Design review of the part shown in the three views and the two pictorial views. Dimensions are in mm from the part's minimum x, y and z. A direction names the side the tool comes from. Give positions to 0.01 mm unless a question says otherwise; leave off trailing zeros. Order: outer loops, then holes, each group sorted by start corner. A loop starts at its lowest first (then second) coordinate and runs counter-clockwise, first axis right, second up.
Item 1: Consider section D-D (z = 32.5). Give the boundary of the cut face in (x, y), plus the area to 3 significant figures.
Item 2: For probe 1 along X at (y, z) = (17, 41); probe 2 along Z at (x, y) = (9, 12.5); probe 3 along X at (y, z) = (16.25, 16), list the stretches that pass through material, from the lowest coordinate up.
Item 3: The part is to be moulded in two halves that separate along Z. For the marked faces 1, 2, 3 and 4, say which applies: released by +Z, released by -Z, zero draft, split by the parting line, or undercut.
Item 4: Machinability: for the marked faces 5, 6, 7 and 8, which of the approach directions +Z, -Z, +X, -X, +Y, -Y give a long, thin tool a straight path to every point of the face, cutting with its end or side? Answer none if there is none.
Item 5: For P1, Ø5, axis at x = 43, y = 2, coming from the -Z side; P2, Ø6, axis at y = 8.5, z = 53.5, coming from the +X side; P3, Ø3, axis at x = 6.5, z = 18, coming from the -Y side; P4, Ø6, axis at y = 9, z = 29.5, coming from the -X side, all flat-tipped, find the tip position at first contact; note any pin that passes through.
Item 6: Consider section C-C (x = 7.5). Give the boundary of the cut face in (y, z), plus the area to 3 significant figures.
Item 7: Consider section A-A (y = 7.5). Give the number of separate pieces and of enclosed holes in the cut face, plus the area to 4 significant figures.
Item 8: Consider section B-B (z = 44). Give the boundary of the cut face in (x, y), plus the area to 3 significant figures.
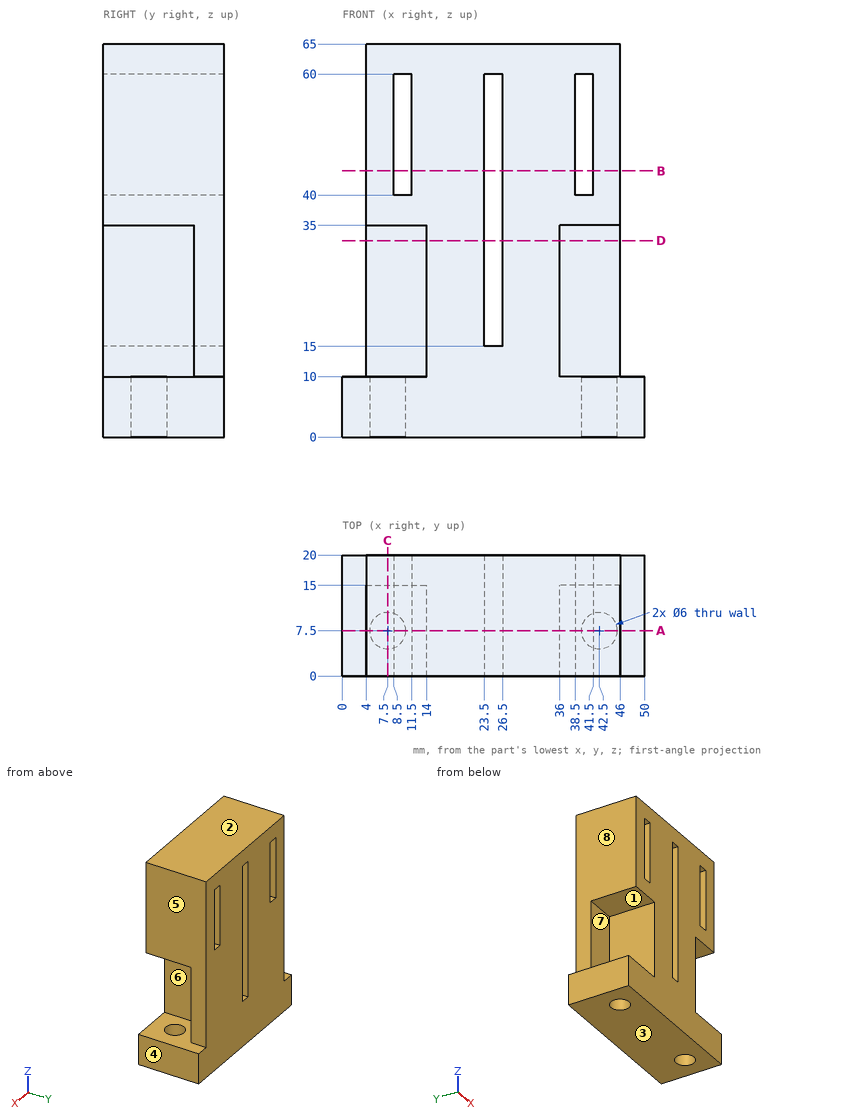
Resolved:
1. outline: (4, 15) - (14, 15) - (14, 0) - (23.5, 0) - (23.5, 20) - (4, 20) - close; (26.5, 0) - (36, 0) - (36, 15) - (46, 15) - (46, 20) - (26.5, 20) - close
1. area: 480 mm2
2. probe 1: x = 4 to 8.5, 11.5 to 23.5, 26.5 to 38.5, 41.5 to 46
2. probe 2: z = 0 to 10, 35 to 40, 60 to 65
2. probe 3: x = 4 to 23.5, 26.5 to 46
3. face 1: undercut
3. face 2: released by +Z
3. face 3: released by -Z
3. face 4: zero draft
4. face 5: +Z, +X, +Y, -Y
4. face 6: +X, -Y
4. face 7: -X, -Y
4. face 8: +Z, -X, +Y, -Y
5. P1: stops at z = 0
5. P2: stops at x = 46
5. P3: stops at y = 15
5. P4: stops at x = 14
6. outline: (0, 0) - (4.5, 0) - (4.5, 10) - (0, 10) - close; (0, 35) - (15, 35) - (15, 10) - (10.5, 10) - (10.5, 0) - (20, 0) - (20, 65) - (0, 65) - close
6. area: 865 mm2
7. separate pieces: 3
7. enclosed holes: 3
7. area: 1,935 mm2
8. outline: (4, 0) - (8.5, 0) - (8.5, 20) - (4, 20) - close; (11.5, 0) - (23.5, 0) - (23.5, 20) - (11.5, 20) - close; (26.5, 0) - (38.5, 0) - (38.5, 20) - (26.5, 20) - close; (41.5, 0) - (46, 0) - (46, 20) - (41.5, 20) - close
8. area: 660 mm2
